```python
from build123d import *

# Parameters (mm, degrees)
F0_W     = 65.023827
F0_H     = 50
F1_DEPTH = 25
F2_R     = 9
F3_DEPTH = 25.001
F4_R     = 17.5
F5_DEPTH = 2
F6_R     = 4


with BuildPart() as f1:
    # F0 (on Top) → F1 (new body)
    with BuildSketch(Plane.XY):
        with Locations((8.511913, 0)):
            Rectangle(F0_W, F0_H)
    extrude(amount=-F1_DEPTH)

    # F2 (on face) → F3 (cut, through all)
    with BuildSketch(Plane.XY):
        Circle(F2_R)
    extrude(amount=-F3_DEPTH, mode=Mode.SUBTRACT)

    # F4 (on face) → F5 (cut)
    with BuildSketch(Plane.XY):
        Circle(F4_R)
    extrude(amount=-F5_DEPTH, mode=Mode.SUBTRACT)

    # F6
    f6_edges = [f1.edges().sort_by_distance(p)[0] for p in [
        (-24, 0, 0),
    ]]
    fillet(f6_edges, radius=F6_R)


solid = f1.part
```
The listing builds one solid part. Answer for the finished solid, in the listing's coordinates (mm). A direction names the side the tool comes from. Round coordinates to 2 decimals unless told otherwise and drop trailing zeros. Loops run counter-clockwise (first coordinate to the right, second up) from the corner with the lowest first, then second, coordinate; pieces in that order, holes last.
Q1. For a pull along Y with two mould halves and no side action, classify faces 1 (the face through (-13.887, -10.648, -0.986)), 2 (the face through (8, 25, -12)), 3 (the face through (8, -25, -12)), 4 (the face through (8, 6, -25)) as released by +Y, released by -Y, zero draft, split by the parting line, or undercut.
Q2. Which of the six approach directions +Z, -Z, +X, -X, +Y, -Y give full straight-line access (tool end or side, diameter ignored) to faces 5 (the face through (8, -8, -2)), 6 (the face through (41.024, 0, -12))?
Q3. Section C-C, the plane z = -17.5 is taken. Determine the outline of the cut face in (x, y).
Q4. Given pin 1 Ø10.5 at (x, y) = (-7.5, -7) entering from +Z, flat-ended and moving along its own axis, determine where the tip first touches the part or whether it passes through.
Q5. Section A-A, the plane x = 0 is taken. Determine the outline of the cut face in (y, z), then the cut area to 3 significant figures.
Q6. Section B-B, the plane y = 0 is taken. Determine the outline of the cut face in (x, z).
Q7. Section D-D, the plane y = 13 is taken. Determine the outline of the cut face in (x, z), then the cut area to 3 significant figures.
Q8. Find the intervals of material crossed by line 1 (Y direction, x = 0, z = -1.5); line 2 (Y direction, x = 0, z = -18.25); line 3 (Z direction, x = -10.5, y = -12), in increasing order.
Completed:
1. face 1: undercut
1. face 2: released by +Y
1. face 3: released by -Y
1. face 4: zero draft
2. face 5: +Z
2. face 6: +Z, -Z, +X, +Y, -Y
3. outline: (-24, -25) - (41.02, -25) - (41.02, 25) - (-24, 25) - close; hole circle Ø18 at (0, 0)
4. pin 1: stops at z = -2
5. outline: (-25, -25) - (-9, -25) - (-9, -2) - (-17.5, -2) - (-17.5, 0) - (-25, 0) - close; (9, -25) - (25, -25) - (25, 0) - (17.5, 0) - (17.5, -2) - (9, -2) - close
5. area: 766 mm2
6. outline: (-24, -25) - (-9, -25) - (-9, -2) - (-17.5, -2) - (-17.5, 0) - (-20, 0) arc R4 ccw to (-24, -4) - close; (9, -25) - (41.02, -25) - (41.02, 0) - (17.5, 0) - (17.5, -2) - (9, -2) - close
7. outline: (-24, -25) - (41.02, -25) - (41.02, 0) - (11.72, 0) - (11.72, -2) - (-11.72, -2) - (-11.72, 0) - (-20, 0) arc R4 ccw to (-24, -4) - close
7. area: 1,580 mm2
8. line 1: y = -25 to -17.5, 17.5 to 25
8. line 2: y = -25 to -9, 9 to 25
8. line 3: z = -25 to -2
